from build123d import *

# Parameters (mm, degrees)
SKETCH_1_W      = 15
SKETCH_1_H      = 11
EXTRUDE_1_DEPTH = 2
SKETCH_2_W      = 4
SKETCH_2_H      = 5
EXTRUDE_2_DEPTH = 1
SKETCH_3_W      = 2
SKETCH_3_H      = 7.956602162
EXTRUDE_3_DEPTH = 2


with BuildPart() as part:
    # 스케치1 → 보스-돌출1 (new body)
    with BuildSketch(Plane(origin=(0, 0, 0), x_dir=(1, 0, 0), z_dir=(0, 1, 0))):
        Rectangle(SKETCH_1_W, SKETCH_1_H)
    extrude(amount=EXTRUDE_1_DEPTH)

    # 스케치2 → 보스-돌출2 (add)
    with BuildSketch(Plane(origin=(0, 2, 0), x_dir=(1, 0, 0), z_dir=(0, 1, 0))):
        with Locations((5, 0)):
            Rectangle(SKETCH_2_W, SKETCH_2_H)
    extrude(amount=EXTRUDE_2_DEPTH)

    # 스케치3 → 보스-돌출3 (add)
    with BuildSketch(Plane.XZ):
        with Locations((-6.098780992, 0)):
            Rectangle(SKETCH_3_W, SKETCH_3_H)
    extrude(amount=EXTRUDE_3_DEPTH)


solid = part.part
Design review of the part built by this model. Coordinates are the model's own, in mm. A direction names the side the tool comes from. Coordinates: 2 decimals unless noted, no trailing zeros. Order: outer loops, then holes, each group sorted by start corner. A loop starts at its lowest first (then second) coordinate and runs counter-clockwise, first axis right, second up. Notation, with made-up numbers: M -9,87 L 17,87 A15 ccw 17,109 Z; hole C 67,47.25 d6. An arc over 180 degrees is marked long. Use a Markdown table: item, result.
(1) Add section C-C (y = -0.4). Give the boundary of the cut face in (x, z), then the cut area to 3 significant figures.
Worked answers:
| item | result |
|---|---|
| outline | M -7.1,-3.98 L -5.1,-3.98 L -5.1,3.98 L -7.1,3.98 Z |
| area | 15.9 mm2 |
(2) Wall thickness on probe 1 along Y at (x, z) = (-2.75, 0.5); probe 2 along X at (y, z) = (-1.3, 3.25); probe 3 along X at (y, z) = (2.7, -0.25): over which ranges is each line inside the solid? List them lowest first.
Worked answers:
| item | result |
|---|---|
| probe 1 | y = 0 to 2 |
| probe 2 | x = -7.1 to -5.1 |
| probe 3 | x = 3 to 7 |
(3) Add section D-D (z = 2). Give the boundary of the cut face in (x, y).
Worked answers:
| item | result |
|---|---|
| outline | M -7.5,0 L -7.1,0 L -7.1,-2 L -5.1,-2 L -5.1,0 L 7.5,0 L 7.5,2 L 7,2 L 7,3 L 3,3 L 3,2 L -7.5,2 Z |
(4) For faces 1 (the flat face through (3, 2.5, 0)), 2 (the flat face through (5, 2.5, -2.5)), 3 (the flat face through (-6, -1, -3.978)), 4 (the flat face through (-5.099, -1, 0)), 5 (the flat face through (-7.099, -1, 0)), list the 3-axis set-ups (+Z, -Z, +X, -X, +Y, -Y) from which the entire face can be reached by the end or side of a thin tool; tool diameter is ignored.
Worked answers:
| item | result |
|---|---|
| face 1 | +Z, -Z, -X, +Y |
| face 2 | -Z, +X, -X, +Y |
| face 3 | -Z, +X, -X, -Y |
| face 4 | +Z, -Z, +X, -Y |
| face 5 | +Z, -Z, -X, -Y |
(5) Add section B-B (x = 5.25). Give the boundary of the cut face in (y, z), then the cut area to 3 significant figures.
Worked answers:
| item | result |
|---|---|
| outline | M 0,-5.5 L 2,-5.5 L 2,-2.5 L 3,-2.5 L 3,2.5 L 2,2.5 L 2,5.5 L 0,5.5 Z |
| area | 27.0 mm2 |
(6) Add section A-A (z = 3.5). Give the boundary of the cut face in (x, y).
Worked answers:
| item | result |
|---|---|
| outline | M -7.5,0 L -7.1,0 L -7.1,-2 L -5.1,-2 L -5.1,0 L 7.5,0 L 7.5,2 L -7.5,2 Z |
(7) For P1, Ø6, axis at x = 1, z = -3.5, coming from the -Y side; P2, Ø0.6, axis at x = -6, y = -1, coming from the +Z side; P3, Ø1, axis at x = -6, y = -1, coming from the -Z side, all flat-tipped, find the tip position at first contact; note any pin that passes through.
Worked answers:
| item | result |
|---|---|
| P1 | stops at y = 0 |
| P2 | stops at z = 3.98 |
| P3 | stops at z = -3.98 |
